Read the model definition and answer for the solid it produces. Units are mm, in the model's axes. A direction names the side the tool comes from. Give positions to 0.01 mm unless a question says otherwise; leave off trailing zeros. Loops run counter-clockwise (first coordinate to the right, second up) from the corner with the lowest first, then second, coordinate; pieces in that order, holes last. Notation, with made-up numbers: (41, 24) - (76, 24) arc R28 cw to (76, 45) - close; hole circle Ø7 at (52, 47.5). An arc over 180 degrees is marked (long way). Write each question's results on one line, items separated by ' | '. Start each with the question number.
Q1. For faces 5 (the flat face through (1, 12.7, 25)), 6 (the flat face through (15.875, 15, 68)), 7 (the flat face through (6, 6, 15.24)), determine the directions among +Z, -Z, +X, -X, +Y, -Y from which every point of the face is accessible in a straight line to the end or side of a thin tool.
Q2. The part is cut by section C-C, the plane x = 6.35. Write down the section's boundary in (y, z), plus the area to 3 significant figures.
Q3. Determine the mould class of faces 1 (the flat face through (-11, 25.4, 75)), 2 (the cylindrical face through (2.84, 3.13, 6.26)), 3 (the flat face through (-3.175, 15, 68)), 4 (the flat face through (6, 0, 19)) for opening direction Y: +Y half, -Y half, draft (parallel to the pull), parting line (faces both ways), or undercut.
Q4. Find the intervals of material crossed by line 1 (Y direction, x = 6.35, z = 9.75); line 2 (Z direction, x = 6.35, y = 3.2); line 3 (X direction, y = 12.5, z = 38.5) (3 decimals), in increasing order. Write a range as from..to.
Q5. Given pin 1 (1 mm diameter, centred on x = -14, z = 41.5, fed in from +Y); pin 2 (12.5 mm diameter, centred on x = -13.5, z = 66, fed in from -Y); pin 3 (5.5 mm diameter, centred on x = 6.35, y = 6.35, fed in from +Z), each flat-ended and moving along its own axis, determine where each tip first touches the part or whether it passes through.
Q6. The part is cut by section B-B, the plane y = 22.75. Write down the section's boundary in (x, z) (3 decimals).
Autodesk Inventor part; units mm, degrees
ref_plane "YZ Plane" through (0, 0, 0) normal (1, 0, 0) x (0, 1, 0)
ref_plane "XZ Plane" through (0, 0, 0) normal (0, 1, 0) x (-1, 0, 0)
ref_plane "XY Plane" through (0, 0, 0) normal (0, 0, 1) x (1, 0, 0)
sketch "Sketch1" plane through (0, 0, 0) normal (0, 0, 1) x (1, 0, 0)
  line L0 (0, 0) -> (12.7, 0)
  line L1 (12.7, 0) -> (12.7, 12.7)
  line L2 (12.7, 12.7) -> (0, 12.7)
  line L3 (0, 12.7) -> (0, 0)
  circle A0 centre (6.35, 6.35) radius 4.7625
  dimension "d0" = 12.7
  dimension "d1" = 12.7
  dimension "d2" = 9.525
extrude "Extrusion1" add sketch "Sketch1" along normal blind 12.7
sketch "Sketch2" plane through (0, 0, 12.7) normal (0, 0, 1) x (1, 0, 0)
  line L0 (12.7, 12.7) -> (0, 12.7)
  line L1 (0, 12.7) -> (-19.05, 12.7)
  line L2 (0, 12.7) -> (31.75, 12.7)
  line L3 (31.75, 12.7) -> (31.75, 0)
  line L4 (31.75, 0) -> (-19.05, 0)
  line L5 (-19.05, 0) -> (-19.05, 12.7)
  line L6 (-3.175, 7.9375) -> (15.875, 7.9375)
  line L7 (-3.175, 4.7625) -> (15.875, 4.7625)
  line L8 (15.875, 7.9375) -> (15.875, 4.7625)
  line L9 (-3.175, 7.9375) -> (-3.175, 4.7625)
  point P0 (0, 0)
  dimension "d5" = 19.05
  dimension "d6" = 31.75
extrude "Extrusion2" add sketch "Sketch2" along normal blind 19.05
sketch "Sketch3" plane through (0, 0, 12.7) normal (0, 0, 1) x (1, 0, 0)
  line L0 (-3.175, 7.9375) -> (15.875, 7.9375)
  line L1 (15.875, 4.7625) -> (-3.175, 4.7625)
  line L2 (-3.175, 7.9375) -> (15.875, 7.9375)
  line L3 (15.875, 7.9375) -> (15.875, 4.7625)
  line L4 (15.875, 4.7625) -> (-3.175, 4.7625)
  line L5 (-3.175, 4.7625) -> (-3.175, 7.9375)
  point P0 (0, 0)
extrude "Extrusion3" add sketch "Sketch3" along normal blind 2.54
sketch "Sketch4" plane through (0, 12.7, 0) normal (0, 1, 0) x (1, 0, 0)
  line L0 (-3.175, -31.75) -> (15.875, -31.75)
  line L1 (6.35, -31.75) -> (6.35, -23.4188) construction
  circle A0 centre (6.35, -23.4188) radius 2.5797
  point P0 (0, 0)
  dimension "d15" = 8.3312
  dimension "d16" = 5.1594
extrude "Extrusion4" cut sketch "Sketch4" against normal blind 20.0025
sketch "Sketch5" plane through (0, 0, 31.75) normal (0, 0, 1) x (1, 0, 0)
  line L0 (-3.175, 4.7625) -> (-3.175, 7.9375)
  line L1 (-19.05, 12.7) -> (-19.05, 0)
  line L2 (-3.175, 7.9375) -> (-19.05, 7.9375)
  line L3 (-19.05, 7.9375) -> (-19.05, 12.7)
  line L4 (-19.05, 12.7) -> (-3.175, 12.7)
  line L5 (-3.175, 12.7) -> (-3.175, 7.9375)
  line L6 (-3.175, 7.9375) -> (15.875, 7.9375)
  line L7 (31.75, 12.7) -> (-19.05, 12.7)
  line L8 (15.875, 7.9375) -> (31.75, 7.9375)
  line L9 (31.75, 7.9375) -> (31.75, 12.7)
  line L10 (31.75, 12.7) -> (15.875, 12.7)
  line L11 (15.875, 12.7) -> (15.875, 7.9375)
  point P0 (0, 0)
extrude "Extrusion5" add sketch "Sketch5" along normal blind 50.8 contours L4 L5 L2 L1 | L7 L9 L8 L11
sketch "Sketch6" plane through (0, 12.7, 0) normal (0, 1, 0) x (1, 0, 0)
  line L0 (-3.175, -82.55) -> (-19.05, -82.55)
  line L1 (-3.175, -82.55) -> (-19.05, -82.55)
  line L2 (-19.05, -82.55) -> (-19.05, -66.675)
  line L3 (-19.05, -66.675) -> (-3.175, -66.675)
  line L4 (-3.175, -66.675) -> (-3.175, -82.55)
  line L5 (31.75, -12.7) -> (31.75, -82.55)
  line L6 (15.875, -31.75) -> (15.875, -82.55)
  line L7 (31.75, -82.55) -> (15.875, -82.55)
  line L8 (15.875, -82.55) -> (15.875, -66.675)
  line L9 (15.875, -66.675) -> (31.75, -66.675)
  line L10 (31.75, -66.675) -> (31.75, -82.55)
  point P0 (0, 0)
  dimension "d21" = 15.875
  dimension "d22" = 15.875
extrude "Extrusion6" add sketch "Sketch6" along normal blind 12.7
properties part number "3D Printed Y-piece"
Check sheet entries:
1) face 5: -Z, +X, -X, +Y | face 6: +Z, +Y, -Y | face 7: +Z
2) outline: (0, 0) - (1.59, 0) - (1.59, 12.7) - (11.11, 12.7) - (11.11, 0) - (12.7, 0) - (12.7, 20.84) - (7.94, 20.84) - (7.94, 15.24) - (4.76, 15.24) - (4.76, 20.84) - (0, 20.84) - close; (0, 26) - (4.76, 26) - (4.76, 31.75) - (0, 31.75) - close; (7.94, 26) - (12.7, 26) - (12.7, 31.75) - (7.94, 31.75) - close | area: 181 mm^2
3) face 1: +Y half | face 2: undercut | face 3: draft | face 4: -Y half
4) line 1: y = 0..1.59, 11.11..12.7 | line 2: z = 12.7..20.84, 26..31.75 | line 3: x = -19.05..-3.175, 15.875..31.75
5) pin 1: stops at y = 12.7 | pin 2: stops at y = 7.94 | pin 3: stops at z = 31.75
6) outline: (-19.05, 66.675) - (-3.175, 66.675) - (-3.175, 82.55) - (-19.05, 82.55) - close; (15.875, 66.675) - (31.75, 66.675) - (31.75, 82.55) - (15.875, 82.55) - close
